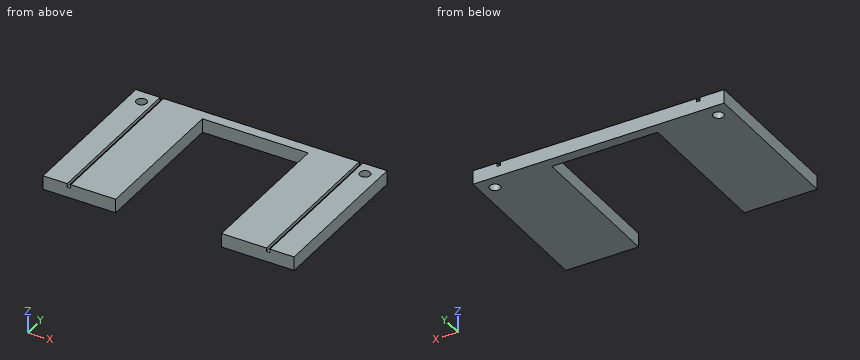
from build123d import *

# Parameters (mm, degrees)
SKETCH1_W           = 72.6
SKETCH1_H           = 45.5
SKETCH1_R           = 1.5
BOSS_EXTRUDE1_DEPTH = 4
SKETCH2_W           = 1
SKETCH2_H           = 45.5
CUT_EXTRUDE1_DEPTH  = 1
SKETCH3_W           = 30.575
SKETCH3_H           = 42.5
CUT_EXTRUDE2_DEPTH  = 4


with BuildPart() as part:
    # Sketch1 → Boss-Extrude1 (new body)
    with BuildSketch(Plane.XY):
        with Locations((36.3, 22.75)):
            Rectangle(SKETCH1_W, SKETCH1_H)
        with Locations((4, 41.5)):
            Circle(SKETCH1_R, mode=Mode.SUBTRACT)
        with Locations((68.6, 41.5)):
            Circle(SKETCH1_R, mode=Mode.SUBTRACT)
    extrude(amount=BOSS_EXTRUDE1_DEPTH)

    # Sketch2 → Cut-Extrude1 (cut)
    with BuildSketch(Plane.XY.offset(4)):
        with Locations((7.5, 22.75)):
            Rectangle(SKETCH2_W, SKETCH2_H)
        with Locations((65.1, 22.75)):
            Rectangle(SKETCH2_W, SKETCH2_H)
    extrude(amount=-CUT_EXTRUDE1_DEPTH, mode=Mode.SUBTRACT)

    # Sketch3 → Cut-Extrude2 (cut)
    with BuildSketch(Plane.XY.offset(4)):
        with Locations((36.3, 21.25)):
            Rectangle(SKETCH3_W, SKETCH3_H)
    extrude(amount=-CUT_EXTRUDE2_DEPTH, mode=Mode.SUBTRACT)


solid = part.part
Input: part model. Units: mm. Frame: model coordinates. Give positions to 0.01 mm unless a question says otherwise; leave off trailing zeros. Write each loop counter-clockwise with the first axis right and the second up, starting at its lowest first coordinate (ties: lowest second). Pieces come first, ordered by that corner, then holes.
Q1. Section B-B, the plane x = 4. Output: boundary loops of the cut face in (y, z), plus the area to 3 significant figures.
Q2. First-contact query: P1, Ø2.5, axis at x = 68.6, y = 41.5, coming from the +Z side; P2, Ø6, axis at x = 64, y = 35, coming from the -Z side; P3, Ø1.2, axis at x = 38, z = 2.5, coming from the -Y side. Flat tips, straight axial feed; report the tip coordinate or a pass-through.
Q3. Section D-D, the plane y = 4.5. Output: boundary loops of the cut face in (x, z), plus the area to 3 significant figures.
Q4. Section C-C, the plane z = 0.95. Output: boundary loops of the cut face in (x, y), plus the area to 3 significant figures.
Q5. Section A-A, the plane y = 41.5. Output: boundary loops of the cut face in (x, z).
Q6. Material intervals for probe 1 along X at (y, z) = (5, 3.45); probe 2 along Y at (x, z) = (68.6, 1.9); probe 3 along X at (y, z) = (26, 0.95), sorted ascending.
Filled in:
1. outline: (0, 0) - (40, 0) - (40, 4) - (0, 4) - close; (43, 0) - (45.5, 0) - (45.5, 4) - (43, 4) - close
1. area: 170 mm2
2. P1: passes through
2. P2: stops at z = 0
2. P3: stops at y = 42.5
3. outline: (0, 0) - (21.01, 0) - (21.01, 4) - (8, 4) - (8, 3) - (7, 3) - (7, 4) - (0, 4) - close; (51.59, 0) - (72.6, 0) - (72.6, 4) - (65.6, 4) - (65.6, 3) - (64.6, 3) - (64.6, 4) - (51.59, 4) - close
3. area: 166 mm2
4. outline: (0, 0) - (21.01, 0) - (21.01, 42.5) - (51.59, 42.5) - (51.59, 0) - (72.6, 0) - (72.6, 45.5) - (0, 45.5) - close; hole circle Ø3 at (4, 41.5); hole circle Ø3 at (68.6, 41.5)
4. area: 1,990 mm2
5. outline: (0, 0) - (2.5, 0) - (2.5, 4) - (0, 4) - close; (5.5, 0) - (21.01, 0) - (21.01, 4) - (8, 4) - (8, 3) - (7, 3) - (7, 4) - (5.5, 4) - close; (51.59, 0) - (67.1, 0) - (67.1, 4) - (65.6, 4) - (65.6, 3) - (64.6, 3) - (64.6, 4) - (51.59, 4) - close; (70.1, 0) - (72.6, 0) - (72.6, 4) - (70.1, 4) - close
6. probe 1: x = 0 to 7, 8 to 21.01, 51.59 to 64.6, 65.6 to 72.6
6. probe 2: y = 0 to 40, 43 to 45.5
6. probe 3: x = 0 to 21.01, 51.59 to 72.6
